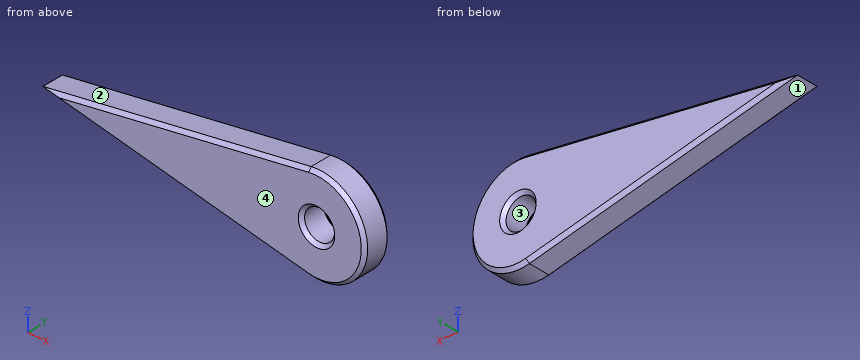
Autodesk Inventor part; units mm, degrees
ref_plane "YZ Plane" through (0, 0, 0) normal (1, 0, 0) x (0, 1, 0)
ref_plane "XZ Plane" through (0, 0, 0) normal (0, 1, 0) x (-1, 0, 0)
ref_plane "XY Plane" through (0, 0, 0) normal (0, 0, 1) x (1, 0, 0)
sketch "Boceto1" plane through (0, 0, 0) normal (0, 1, 0) x (-1, 0, 0)
  circle A0 centre (0, 0) radius 2.7
  arc A1 (1.5138, 8.5673) -> (1.5138, -8.5673) centre (0, 0) ccw
  line L0 (1.5138, 8.5673) -> (50, 0)
  line L1 (50, 0) -> (1.5138, -8.5673)
  dimension "d0" = 5.4
  dimension "d1" = 6
  dimension "d2" = 50
extrude "Extrusión1" add sketch "Boceto1" along normal blind 5
chamfer "Chaflán1" distance 0.6 angle 45 8 edges at (-25.7569, 5, 4.2836) (8.7, 5, 0) (-25.7569, 5, -4.2836) (-25.7569, 0, 4.2836) (8.7, 0, 0) (-25.7569, 0, -4.2836) (2.7, 5, 0) (2.7, 0, 0)
Source: CAD feature listing. Evaluate the final solid. Frame: model axes, mm. Face numbers are marked on the shaded views. Give positions to 0.01 mm unless a question says otherwise; leave off trailing zeros. Write each loop counter-clockwise with the first axis right and the second up, starting at its lowest first coordinate (ties: lowest second). Pieces come first, ordered by that corner, then holes.
1. First-contact query: pin 1 (2 mm diameter, centred on y = 0.5, z = 3.5, fed in from +X). Flat tip, straight axial feed; report the tip coordinate or a pass-through.
2. Section query D-D (x = -26.5). Return the cut outline in (y, z).
3. Section query B-B (x = -7). Return the cut outline in (y, z).
4. Material intervals for line 1 along Z through (x, y) = (0, 1.65); line 2 along Z through (x, y) = (-32, 3.45); line 3 along Z through (x, y) = (6.5, 2.9), sorted ascending.
5. Section query A-A (x = 0). Return the cut outline in (y, z), then the cut area to 3 significant figures.
6. Section query C-C (y = 3). Return the cut outline in (x, z).
7. Pull-direction query (Z, two-part tool) for the marked faces 1, 2, 3 and 4; classes: +Z half, -Z half, draft (parallel to the pull), parting line (faces both ways), or undercut.
Output values:
1. pin 1: stops at x = 8.33
2. outline: (0, -3.54) - (0.6, -4.15) - (4.4, -4.15) - (5, -3.54) - (5, 3.54) - (4.4, 4.15) - (0.6, 4.15) - (0, 3.54) - close
3. outline: (0, -6.99) - (0.6, -7.6) - (4.4, -7.6) - (5, -6.99) - (5, 6.99) - (4.4, 7.6) - (0.6, 7.6) - (0, 6.99) - close
4. line 1: z = -8.7 to -2.7, 2.7 to 8.7
4. line 2: z = -3.18 to 3.18
4. line 3: z = -5.78 to 5.78
5. outline: (0, -8.1) - (0.6, -8.7) - (4.4, -8.7) - (5, -8.1) - (5, -3.3) - (4.4, -2.7) - (0.6, -2.7) - (0, -3.3) - close; (0, 3.3) - (0.6, 2.7) - (4.4, 2.7) - (5, 3.3) - (5, 8.1) - (4.4, 8.7) - (0.6, 8.7) - (0, 8.1) - close
5. area: 58.6 mm2
6. outline: (-50, 0) - (-1.51, -8.57) arc R8.7 ccw (long way) to (-1.51, 8.57) - close; hole circle Ø5.4 at (0, 0)
7. face 1: -Z half
7. face 2: +Z half
7. face 3: undercut
7. face 4: draft
